from build123d import *

# Parameters (mm, degrees)
F0_W     = 59
F0_H     = 41
F1_DEPTH = 21
F2_R     = 3
F3_R     = 10.5
F4_DEPTH = 7


with BuildPart() as f1:
    # F0 (on Top) → F1 (new body)
    with BuildSketch(Plane.XY):
        Rectangle(F0_W, F0_H)
    extrude(amount=F1_DEPTH)

    # F2
    f2_edges = [f1.edges().sort_by_distance(p)[0] for p in [
        (-29.5, -20.5, 10.5),
        (-29.5, 20.5, 10.5),
        (29.5, -20.5, 10.5),
        (29.5, 20.5, 10.5),
    ]]
    fillet(f2_edges, radius=F2_R)

    # F3 (on face) → F4 (join)
    with BuildSketch(Plane.XY.offset(21)):
        with Locations((16.302584, 7.747762)):
            Circle(F3_R)
    extrude(amount=F4_DEPTH)


solid = f1.part
For this review, take the finished solid that the model builds, in its own axes (mm). A direction names the side the tool comes from. Give positions to 0.01 mm unless a question says otherwise; leave off trailing zeros. Order: outer loops, then holes, each group sorted by start corner. A loop starts at its lowest first (then second) coordinate and runs counter-clockwise, first axis right, second up. Notation, with made-up numbers: (-38, 53) - (-3, 53) arc R12 ccw to (-3, 65) - close; hole circle Ø10 at (-17.75, 66). An arc over 180 degrees is marked (long way). Answer as a JSON object with one key per item and string values. Group by question number.
Item 1: Take a section at C-C on z = 24.5. Give the boundary of the cut face in (x, y).
Item 2: Take a section at D-D on x = -21.5. Give the boundary of the cut face in (y, z).
Item 3: Take a section at B-B on y = -7.5. Give the boundary of the cut face in (x, z).
Item 4: Machinability: for faces 1 (the cylindrical face through (8.56, 14.84, 24.45)), 2 (the cylindrical face through (-28.64, 19.6, 10.65)), which of the approach directions +Z, -Z, +X, -X, +Y, -Y give a long, thin tool a straight path to every point of the face, cutting with its end or side? Answer none if there is none.
Item 5: Take a section at A-A on x = 16. Give the boundary of the cut face in (y, z).
Item 6: Wall thickness on line 1 along Z through (x, y) = (-5, -9); line 2 along Y through (x, z) = (17.5, 26.25); line 3 along X through (y, z) = (13.5, 23.5): over which ranges is each line inside the solid? List them lowest first.
Reported:
{
 "1": {"outline": "circle Ø21 at (16.3, 7.75)"},
 "2": {"outline": "(-20.5, 0) - (20.5, 0) - (20.5, 21) - (-20.5, 21) - close"},
 "3": {"outline": "(-29.5, 0) - (29.5, 0) - (29.5, 21) - (-29.5, 21) - close"},
 "4": {"face 1": "+Z", "face 2": "+Z, -Z, -X, +Y"},
 "5": {"outline": "(-20.5, 0) - (20.5, 0) - (20.5, 21) - (18.24, 21) - (18.24, 28) - (-2.75, 28) - (-2.75, 21) - (-20.5, 21) - close"},
 "6": {"line 1": "0 to 21", "line 2": "-2.68 to 18.18", "line 3": "7.52 to 25.09"}
}
